Geometry check sheet. Reference: drawing and pictorial views, mm from the part's lowest x, y, z. A direction names the side the tool comes from. Give positions to 0.01 mm unless a question says otherwise; leave off trailing zeros. Order: outer loops, then holes, each group sorted by start corner. A loop starts at its lowest first (then second) coordinate and runs counter-clockwise, first axis right, second up.
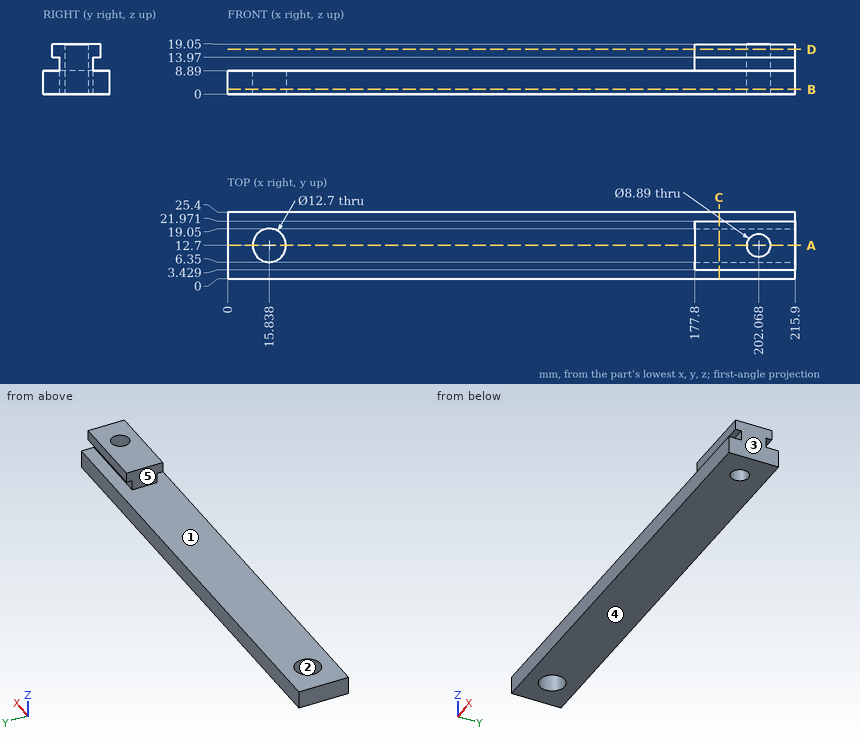
1) Section check D-D, the plane z = 17. Record the cut outline in (x, y) (1 decimal), then the cut area to 3 significant figures.
Recorded:
outline: (177.8, 3.4) - (215.9, 3.4) - (215.9, 22) - (177.8, 22) - close; hole circle Ø8.9 at (202.1, 12.7)
area: 644 mm2
2) Section check A-A, the plane y = 12.7. Record the cut outline in (x, z), then the cut area to 3 significant figures.
Recorded:
outline: (0, 0) - (9.49, 0) - (9.49, 8.89) - (0, 8.89) - close; (22.19, 0) - (197.62, 0) - (197.62, 19.05) - (177.8, 19.05) - (177.8, 8.89) - (22.19, 8.89) - close; (206.51, 0) - (215.9, 0) - (215.9, 19.05) - (206.51, 19.05) - close
area: 2,020 mm2
3) Section check B-B, the plane z = 1.75. State how many separate pieces and enclosed holes the cut face has, then the cut area to 4 significant figures.
Recorded:
separate pieces: 1
enclosed holes: 2
area: 5,295 mm2
4) Depth check by flat-ended pin: pin 1 Ø4 at (y, z) = (20, 8) entering from -X; pin 2 Ø6 at (x, y) = (173, 8) entering from +Z; pin 3 Ø2.5 at (x, z) = (192.5, 11) entering from +Y; pin 4 Ø2.5 at (x, z) = (202.5, 11.5) entering from -Y. Enter the tip coordinate at first touch or a pass-through.
Recorded:
pin 1: stops at x = 0
pin 2: stops at z = 8.89
pin 3: stops at y = 19.05
pin 4: stops at y = 6.35
5) Set-up check for the marked faces 4 and 5: record each of +Z, -Z, +X, -X, +Y, -Y from which the full face is reachable in a straight line by a thin tool's end or side.
Recorded:
face 4: -Z, +X, -X, +Y, -Y
face 5: +Z, -X, +Y, -Y
6) Section check C-C, the plane x = 187. Record the cut outline in (y, z).
Recorded:
outline: (0, 0) - (25.4, 0) - (25.4, 8.89) - (19.05, 8.89) - (19.05, 13.97) - (21.97, 13.97) - (21.97, 19.05) - (3.43, 19.05) - (3.43, 13.97) - (6.35, 13.97) - (6.35, 8.89) - (0, 8.89) - close
7) Material ranges on L1, parallel to X at y = 12.25, z = 3.5; L2, parallel to Z at x = 134, y = 12.25; L3, parallel to X at y = 15, z = 17.75 (1 decimal), recorded low to high.
Recorded:
L1: x = 0 to 9.5, 22.17 to 197.65, 206.49 to 215.9
L2: z = 0 to 8.89
L3: x = 177.8 to 198.3, 205.9 to 215.9
8) Draft check along X on the marked faces 1, 2 and 3. Enter one of: +X half, -X half, draft (parallel to the pull), parting line (faces both ways), or undercut.
Recorded:
face 1: draft
face 2: undercut
face 3: +X half
